Autodesk Inventor part; units mm, degrees
ref_plane "YZ Plane" through (0, 0, 0) normal (1, 0, 0) x (0, 1, 0)
ref_plane "XZ Plane" through (0, 0, 0) normal (0, 1, 0) x (-1, 0, 0)
ref_plane "XY Plane" through (0, 0, 0) normal (0, 0, 1) x (1, 0, 0)
sketch "スケッチ1" plane through (0, 0, 0) normal (0, 0, 1) x (1, 0, 0)
  line L0 (-3.8522, 2.7979) -> (11.1478, 2.7979)
  line L1 (11.1478, 2.7979) -> (11.1478, -27.2021)
  line L2 (11.1478, -27.2021) -> (-3.8522, -27.2021)
  line L3 (-3.8522, -27.2021) -> (-3.8522, 2.7979)
  point P0 (0, 0)
  dimension "d0" = 15
  dimension "d1" = 30
extrude "押し出し1" add sketch "スケッチ1" along normal blind 350
sketch "スケッチ2" plane through (-3.8522, 2.7979, 0) normal (0, 1, 0) x (1, 0, 0)
  circle A0 centre (7.5, -335) radius 1.5
  line L0 (15, -350) -> (0, -350)
  circle A1 centre (7.5, -325) radius 1.5
  circle A2 centre (7.5, -315) radius 1.5
  line L1 (0, 0) -> (0, -350)
  line L2 (15, 0) -> (15, -350)
  circle A3 centre (7.5, -15) radius 1.5
  line L3 (0, 0) -> (15, 0)
  circle A4 centre (7.5, -25) radius 1.5
  circle A5 centre (7.5, -35) radius 1.5
  point P0 (3.8522, 0)
  dimension "d4" = 3
  dimension "d5" = 15
  dimension "d6" = 3
  dimension "d7" = 3
  dimension "d8" = 10
  dimension "d9" = 10
  dimension "d10" = 7.5
  dimension "d11" = 7.5
  dimension "d12" = 7.5
  dimension "d13" = 3
  dimension "d14" = 15
  dimension "d15" = 7.5
  dimension "d16" = 3
  dimension "d17" = 3
  dimension "d18" = 10
  dimension "d19" = 10
hole "穴1" at (3.6478, 2.7979, 335) at (3.6478, 2.7979, 325) at (3.6478, 2.7979, 315) at (3.6478, 2.7979, 35) at (3.6478, 2.7979, 25) at (3.6478, 2.7979, 15) direction (0, -1, 0) diameter 3 depth 30
sketch "スケッチ3" plane through (0, 0, 0) normal (0, 0, -1) x (-1, 0, 0)
  line L0 (-9.6478, 1.2979) -> (2.3522, 1.2979)
  line L1 (2.3522, 1.2979) -> (2.3522, -25.7021)
  line L2 (2.3522, -25.7021) -> (-9.6478, -25.7021)
  line L3 (-9.6478, -25.7021) -> (-9.6478, 1.2979)
  line L4 (3.8522, 2.7979) -> (-11.1478, 2.7979)
  line L5 (-11.1478, 2.7979) -> (-11.1478, -27.2021)
  point P0 (0, 0)
  dimension "d27" = 12
  dimension "d28" = 27
  dimension "d29" = 1.5
  dimension "d30" = 1.5
extrude "押し出し2" cut sketch "スケッチ3" against normal blind 350
sketch "スケッチ4" plane through (-3.8522, 2.7979, 0) normal (0, 1, 0) x (1, 0, 0)
  point P0 (3.8522, 0)
properties part number "nhk9" material "アルミニウム 6061"
Read the model definition and answer for the solid it produces. Units are mm, in the model's axes. A direction names the side the tool comes from. Give positions to 0.01 mm unless a question says otherwise; leave off trailing zeros. Write each loop counter-clockwise with the first axis right and the second up, starting at its lowest first coordinate (ties: lowest second). Pieces come first, ordered by that corner, then holes. Notation, with made-up numbers: (65.25, 15) - (70.25, 15) arc R11 ccw to (70.25, 22) - close; hole circle Ø11 at (1.5, 23.25). An arc over 180 degrees is marked (long way). Answer in a Markdown table with one row per item. Add a question column.
Item 1: A tool of negligible diameter and unlimited length cuts with its end or side. For faces 5 (the face through (9.648, -12, 173)), 6 (the face through (4, 2.798, 173)), from which of +Z, -Z, +X, -X, +Y, -Y can it reach the whole face along a straight path? Write none if from no direction.
Item 2: Determine the mould class of faces 1 (the face through (-2.352, -12, 173)), 2 (the face through (11.148, -12, 173)), 3 (the face through (-3.852, -12, 173)), 4 (the face through (10, -12, 0)) for opening direction X: pulls with the +X half, pulls with the -X half, needs draft (parallel to the pull), parting line crosses it, or undercut.
Item 3: Section A-A, the plane y = -6.5 is taken. Write down the section's boundary in (x, z), and give its area (3 significant figures).
Item 4: A flat-ended cylindrical pin translates along its axis: P1, Ø2.5, axis at x = 3.65, z = 35, coming from the +Y side. Find the tip coordinate at first contact, or state that the pin passes through.
Item 5: Find the intervals of material crossed by L1, parallel to X at y = 2.5, z = 335; L2, parallel to Y at x = 5.5, z = 160.5; L3, parallel to X at y = -7.25, z = 319, in increasing order.
Item 6: Section B-B, the plane z = 108 is taken. Write down the section's boundary in (x, y).
Recorded:
| question | item | result |
|---|---|---|
| 1 | face 5 | +Z, -Z |
| 1 | face 6 | +Z, -Z, +X, -X, +Y |
| 2 | face 1 | undercut |
| 2 | face 2 | pulls with the +X half |
| 2 | face 3 | pulls with the -X half |
| 2 | face 4 | needs draft |
| 3 | outline | (-3.85, 0) - (-2.35, 0) - (-2.35, 350) - (-3.85, 350) - close; (9.65, 0) - (11.15, 0) - (11.15, 350) - (9.65, 350) - close |
| 3 | area | 1,050 mm2 |
| 4 | P1 | passes through |
| 5 | L1 | x = -3.85 to 2.15, 5.15 to 11.15 |
| 5 | L2 | y = -27.2 to -25.7, 1.3 to 2.8 |
| 5 | L3 | x = -3.85 to -2.35, 9.65 to 11.15 |
| 6 | outline | (-3.85, -27.2) - (11.15, -27.2) - (11.15, 2.8) - (-3.85, 2.8) - close; hole (-2.35, -25.7) - (9.65, -25.7) - (9.65, 1.3) - (-2.35, 1.3) - close |
